```python
from build123d import *

# Parameters (mm, degrees)
SKETCH1_R           = 2.1
SKETCH1_R_2         = 5
BOSS_EXTRUDE1_DEPTH = 3
SKETCH3_R           = 1.6
CUT_EXTRUDE1_DEPTH  = 10
FILLET1_R           = 5
SKETCH4_R           = 3
CUT_EXTRUDE2_DEPTH  = 1.5


with BuildPart() as part:
    # Sketch1 → Boss-Extrude1 (new body)
    with BuildSketch(Plane(origin=(0, 0, 0), x_dir=(1, 0, 0), z_dir=(0, 1, 0))):
        with BuildLine():
            Line((-8, 17.5), (-8, -17.5))
            Line((-8, -17.5), (0, -17.5))
            Line((0, -17.5), (32.082434223, -5.627030097))
            ThreePointArc((32.082434223, -5.627030097), (36, 0), (32.082434223, 5.627030097))
            Line((32.082434223, 5.627030097), (0, 17.5))
            Line((0, 17.5), (-8, 17.5))
        make_face()
        with Locations(Location((30, 0, 0), (0, 0, 270))):
            Circle(SKETCH1_R, mode=Mode.SUBTRACT)
        with Locations(Location((0, 0, 0), (0, 0, 270))):
            Circle(SKETCH1_R_2, mode=Mode.SUBTRACT)
    extrude(amount=BOSS_EXTRUDE1_DEPTH)

    # Sketch3 → Cut-Extrude1 (cut)
    with BuildSketch(Plane(origin=(0, 3, 0), x_dir=(1, 0, 0), z_dir=(0, 1, 0))):
        with Locations(Location((0, 13.75, 0), (0, 0, 270))):
            Circle(SKETCH3_R)
        with Locations(Location((11.315438541, 9.754896669, 0), (0, 0, 270))):
            Circle(SKETCH3_R)
        with Locations(Location((22.630877082, 5.759793337, 0), (0, 0, 270))):
            Circle(SKETCH3_R)
        with Locations(Location((22.630877082, -5.759793337, 0), (0, 0, 270))):
            Circle(SKETCH3_R)
        with Locations(Location((0, -13.75, 0), (0, 0, 270))):
            Circle(SKETCH3_R)
        with Locations(Location((11.315438541, -9.754896669, 0), (0, 0, 270))):
            Circle(SKETCH3_R)
    extrude(amount=-CUT_EXTRUDE1_DEPTH, mode=Mode.SUBTRACT)

    # Fillet1
    fillet1_edges = [part.edges().sort_by_distance(p)[0] for p in [
        (-8, 1.5, 17.5),
        (-8, 1.5, -17.5),
    ]]
    fillet(fillet1_edges, radius=FILLET1_R)

    # Sketch4 → Cut-Extrude2 (cut)
    with BuildSketch(Plane(origin=(0, 3, 0), x_dir=(1, 0, 0), z_dir=(0, 1, 0))):
        with Locations(Location((0, 13.75, 0), (0, 0, 270))):
            Circle(SKETCH4_R)
        with Locations(Location((11.315438541, 9.754896669, 0), (0, 0, 270))):
            Circle(SKETCH4_R)
        with Locations(Location((22.630877082, 5.759793337, 0), (0, 0, 270))):
            Circle(SKETCH4_R)
        with Locations(Location((22.630877082, -5.759793337, 0), (0, 0, 270))):
            Circle(SKETCH4_R)
        with Locations(Location((11.315438541, -9.754896669, 0), (0, 0, 270))):
            Circle(SKETCH4_R)
        with Locations(Location((0, -13.75, 0), (0, 0, 270))):
            Circle(SKETCH4_R)
    extrude(amount=-CUT_EXTRUDE2_DEPTH, mode=Mode.SUBTRACT)


solid = part.part
```
For this review, take the finished solid that the model builds, in its own axes (mm). A direction names the side the tool comes from. Round coordinates to 2 decimals unless told otherwise and drop trailing zeros. Write each loop counter-clockwise with the first axis right and the second up, starting at its lowest first coordinate (ties: lowest second). Pieces come first, ordered by that corner, then holes. Notation, with made-up numbers: (39.25, 89.5) -> (58.25, 89.5) arc R23 cw to (58.25, 124.5) -> close; hole circle Ø10 at (9.5, 57). An arc over 180 degrees is marked (long way). One line per question, with ' | ' between items. Start each with the question number.
1) Add section A-A (z = 0). Write out the cut boundary in (x, y), and give its area (3 significant figures).
2) Add section B-B (z = 14). Write out the cut boundary in (x, y), and give its area (3 significant figures).
3) Add section C-C (y = 0.9). Count the separate pieces of the cut face and the enclosed holes in it, and give its area (3 significant figures).
4) Machinability: for faces 1 (the flat face through (-1, 1.5, -12)), 2 (the cylindrical face through (10.342, 0.76, -11.025)), which of the approach directions +Z, -Z, +X, -X, +Y, -Y give a long, thin tool a straight path to every point of the face, cutting with its end or side? Answer none if there is none.
5) Wall thickness on line 1 along X through (y, z) = (1.75, 0); line 2 along Z through (x, y) = (10.5, 2.25); line 3 along Z through (x, y) = (23, 1.15): over which ranges is each line inside the solid? List them lowest first.
6) For pin 1 Ø3 at (x, z) = (22.5, 5.5) entering from +Y, flat-tipped, find the tip position at first contact; note if it passes through.
7) Mouldability with a two-part tool opening along X and no side actions: class faces 3 (the flat face through (21, 1.5, -4)), 4 (the cylindrical face through (9.49, 2.26, -12.136)), 5 (the flat face through (-1, 1, -17.5)), 6 (the flat face through (-8, 1, 0)) as +X half, -X half, draft (parallel to the pull), parting line (faces both ways), or undercut.
8) Add section D-D (x = 30). Write out the cut boundary in (y, z), and give its area (3 significant figures).
Reported:
1) outline: (-8, 0) -> (-5, 0) -> (-5, 3) -> (-8, 3) -> close; (5, 0) -> (27.9, 0) -> (27.9, 3) -> (5, 3) -> close; (32.1, 0) -> (36, 0) -> (36, 3) -> (32.1, 3) -> close | area: 89.4 mm²
2) outline: (-7.77, 0) -> (-1.58, 0) -> (-1.58, 1.5) -> (-2.99, 1.5) -> (-2.99, 3) -> (-7.77, 3) -> close; (1.58, 0) -> (9.46, 0) -> (9.46, 3) -> (2.99, 3) -> (2.99, 1.5) -> (1.58, 1.5) -> close | area: 38.0 mm²
3) separate pieces: 1 | enclosed holes: 8 | area: 903 mm²
4) face 1: +Y | face 2: +Y, -Y
5) line 1: x = -8 to -5, 5 to 27.9, 32.1 to 36 | line 2: z = -13.61 to -12.64, -6.87 to 6.87, 12.64 to 13.61 | line 3: z = -8.99 to -7.32, -4.2 to 4.2, 7.32 to 8.99
6) pin 1: stops at y = 1.5
7) face 3: undercut | face 4: undercut | face 5: draft | face 6: -X half
8) outline: (0, -6.4) -> (3, -6.4) -> (3, -2.1) -> (0, -2.1) -> close; (0, 2.1) -> (3, 2.1) -> (3, 6.4) -> (0, 6.4) -> close | area: 25.8 mm²
